```python
from build123d import *

# Parameters (mm, degrees)
F1_DEPTH = 3.5
F2_R     = 7.058260031
F3_DEPTH = 25
F4_R     = 6.25
F5_DEPTH = 3.3
F6_R     = 6.25
F7_DEPTH = 3.3
F8_R     = 10


with BuildPart() as f1:
    # F0 (on Top) → F1 (new body)
    with BuildSketch(Plane.XY):
        with BuildLine():
            add(Edge.make_bspline(
                [(27.7347816335, 32.9664582942), (21.7968576271, 27.4921287364), (8.5785934713, 15.3075413902), (30.4614719911, 10.0037248917), (42.4955969964, 7.0802345045)],
                knots=[0, 0, 0, 0, 0.4495258402, 1, 1, 1, 1], degree=3))
            ThreePointArc((27.7347816335, 32.9664582942), (-37.424599746, -21.3402159917), (42.4955969964, 7.0802345045))
        make_face()
    extrude(amount=F1_DEPTH)

    # F2 (on Top) → F3 (cut)
    with BuildSketch(Plane.XY):
        with Locations((8.8732391596, 15.4273370281)):
            Circle(F2_R)
    extrude(amount=F3_DEPTH, mode=Mode.SUBTRACT)

    # F4 (on face) → F5 (cut)
    with BuildSketch(Plane.XY.offset(3.5)):
        with Locations((-15.0699157128, 31.2930024222)):
            Circle(F4_R)
        with Locations((-33.8617932364, 7.7287333374)):
            Circle(F4_R)
        with Locations((-28.7774891506, -21.6554295879)):
            Circle(F4_R)
        with Locations((0, -34.7326123432)):
            Circle(F4_R)
        with Locations((27.3688023133, -21.6334286339)):
            Circle(F4_R)
    extrude(amount=-F5_DEPTH, mode=Mode.SUBTRACT)

    # F6 (on face) → F7 (cut)
    with BuildSketch(Plane.XY.offset(3.5)):
        with Locations((-13.9189545551, -10.1127124297)):
            Circle(F6_R)
        with Locations((5.3165675522, -16.3627124297)):
            Circle(F6_R)
        with Locations((-13.9189545551, 10.1127124297)):
            Circle(F6_R)
    extrude(amount=-F7_DEPTH, mode=Mode.SUBTRACT)

    # F8
    f8_edges = [f1.edges().sort_by_distance(p)[0] for p in [
        (27.734782, 32.966458, 1.75),
        (42.495597, 7.080235, 1.75),
    ]]
    fillet(f8_edges, radius=F8_R)


solid = f1.part
```
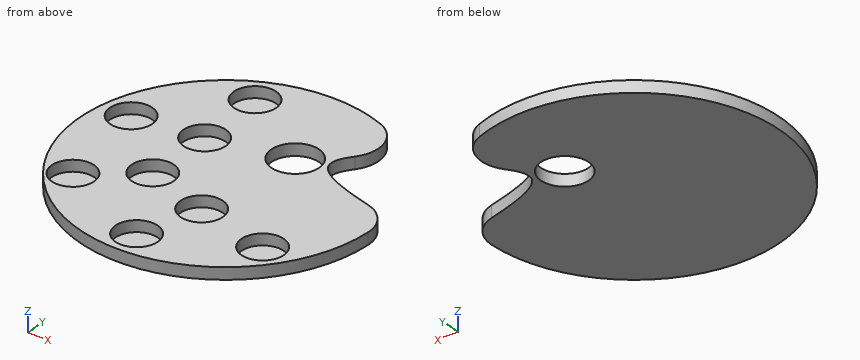
Can you work these out from the model? Positions are in its coordinate system, mm. Coordinates: 2 decimals unless noted, no trailing zeros. Loops run counter-clockwise (first coordinate to the right, second up) from the corner with the lowest first, then second, coordinate; pieces in that order, holes last. Notation, with made-up numbers: (68, 41) - (80, 41) arc R36 cw to (80, 78) - close; hole circle Ø1 at (43.25, -6). An arc over 180 degrees is marked (long way). Answer as CSV lines item,"result". Start each with the question number.
1) For pin 1 (4 mm diameter, centred on x = 30.5, y = -24, fed in from +Z); pin 2 (1.5 mm diameter, centred on y = -12, z = 1, fed in from +X), each with a flat end and sliding along its axis, tell me the tip position at first contact or that it passes through.
2) Suppose I cut it at C-C (x = -29.5). Please give me the cut outline in (y, z).
3) Suppose I cut it at B-B (z = 2.25). Count the separate pieces of the cut face and the enclosed holes in it, plus the area to 3 significant figures.
4) Suppose I cut it at D-D (y = -13). Please give me the cut outline in (x, z).
5) Suppose I cut it at A-A (y = -29.5). Please give me the cut outline in (x, z).
6) I need wall thicknesses on line 1 (X direction, y = 8, z = 0.8); line 2 (X direction, y = 13, z = 0.6); line 3 (Y direction, x = -19, z = 1.95). Which ranges of each line are inside material? Lowest first, please. Write a range as from..to.
Check result:
1,pin 1,"stops at z = 0.2"
1,pin 2,"stops at x = 41.59"
2,outline,"(-31.4, 0) - (31.4, 0) - (31.4, 3.5) - (12.21, 3.5) - (12.21, 0.2) - (3.25, 0.2) - (3.25, 3.5) - (-15.45, 3.5) - (-15.45, 0.2) - (-27.86, 0.2) - (-27.86, 3.5) - (-31.4, 3.5) - close"
3,separate pieces,"1"
3,enclosed holes,"9"
3,area,"4,270 mm²"
4,outline,"(-41.07, 0) - (41.07, 0) - (41.07, 3.5) - (10.58, 3.5) - (10.58, 0.2) - (0.05, 0.2) - (0.05, 3.5) - (-8.38, 3.5) - (-8.38, 0.2) - (-19.46, 0.2) - (-19.46, 3.5) - (-41.07, 3.5) - close"
5,outline,"(-31.4, 0) - (31.4, 0) - (31.4, 3.5) - (3.42, 3.5) - (3.42, 0.2) - (-3.42, 0.2) - (-3.42, 3.5) - (-31.4, 3.5) - close"
6,line 1,"x = -42.33..-40.11, -27.62..-19.8, -8.04..37.66"
6,line 2,"x = -41.07..-37.22, -30.5..-19.46, -8.38..2.25, 15.5..22.66"
6,line 3,"y = -38.67..-13.75, -6.47..6.47, 13.75..26.43, 36.15..38.67"
